Part print with two shaded views. Sizes in mm from the minimum x, y, z corner. A direction names the side the tool comes from. Give positions to 0.01 mm unless a question says otherwise; leave off trailing zeros. Order: outer loops, then holes, each group sorted by start corner. A loop starts at its lowest first (then second) coordinate and runs counter-clockwise, first axis right, second up. Notation, with made-up numbers: M 43.5,-7.75 L 75.5,-7.75 A29 ccw 75.5,29.25 Z; hole C 66.25,74 d9. An arc over 180 degrees is marked long. Return JSON: item names as keys, results as strings.
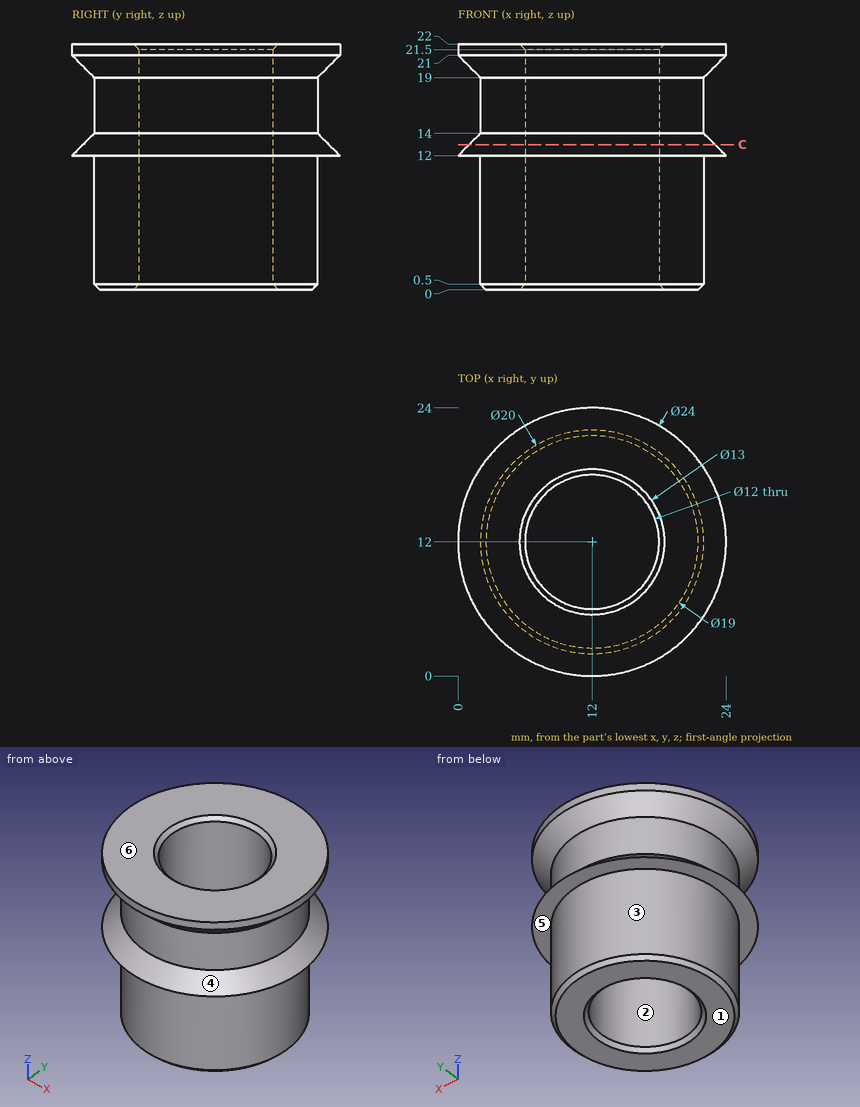
Q1. Band-saw the part on C-C (z = 13). Give the cut face in (x, y).
Established:
{"outline": "C 12,12 d22; hole C 12,12 d12"}
Q2. Pin check, flat tips, straight feed: pin 1 (4 mm diameter, centred on y = 7.5, z = 9.5, fed in from -X); pin 2 (12 mm diameter, centred on y = 10.5, z = 5, fed in from -X); pin 3 (6 mm diameter, centred on y = 20.5, z = 3, fed in from +X). Stop position of each tip, or through.
Established:
{"pin 1": "stops at x = 2.32", "pin 2": "stops at x = 2", "pin 3": "stops at x = 20.35"}
Q3. Probe line 1 along Y through (x, z) = (12, 9.5); line 2 along X through (y, z) = (6.75, 20.75); line 3 along Y through (x, z) = (12, 12.25). List the from-to ranges inside material, lowest first.
Established:
{"line 1": "y = 2 to 6, 18 to 22", "line 2": "x = 1.49 to 9.1, 14.9 to 22.51", "line 3": "y = 0.25 to 6, 18 to 23.75"}
Q4. 3-axis set-ups, long thin cutter, end or side, ignore diameter. For the marked faces 4, 5 and 6: which of +Z, -Z, +X, -X, +Y, -Y reach the whole face in a straight line?
Established:
{"face 4": "none", "face 5": "-Z", "face 6": "+Z, +X, -X, +Y, -Y"}
Q5. Two-plate mould, pull along X, no slides. Class the marked faces 1, 2 and 3: +X half, -X half, draft (parallel to the pull), parting line (faces both ways), or undercut.
Established:
{"face 1": "draft", "face 2": "undercut", "face 3": "parting line"}
